Geometry check sheet. Reference: drawing and pictorial views, mm from the part's lowest x, y, z. Round coordinates to 2 decimals unless told otherwise and drop trailing zeros. Order: outer loops, then holes, each group sorted by start corner. A loop starts at its lowest first (then second) coordinate and runs counter-clockwise, first axis right, second up. Notation, with made-up numbers: (21.5, -5.5) -> (77.5, -5.5) arc R32 ccw to (77.5, 23.5) -> close; hole circle Ø10 at (36, 28.5). An arc over 180 degrees is marked (long way). Return JSON: item names as keys, results as strings. Group by question number.
1) Section check D-D on z = 1.7. Enter the section's corners in (x, y), plus the area to 3 significant figures.
2) Section check A-A on x = 3.25. Enter the section's corners in (y, z), plus the area to 3 significant figures.
3) Section check C-C on y = 0.85. Enter the section's corners in (x, z), plus the area to 3 significant figures.
4) Scan lines: L1, parallel to Z at x = 3.25, y = 0.35; L2, parallel to X at y = 0.3, z = 3.6; L3, parallel to X at y = 0.1, z = 1.85. Record each from-to range of solid material in increasing order.
5) Draft check along X on the marked faces 1 and 2. Enter one of: pulls with the +X half, pulls with the -X half, needs draft (parallel to the pull), parting line crosses it, or undercut.
6) Section check B-B on z = 2.8. Enter the section's corners in (x, y).
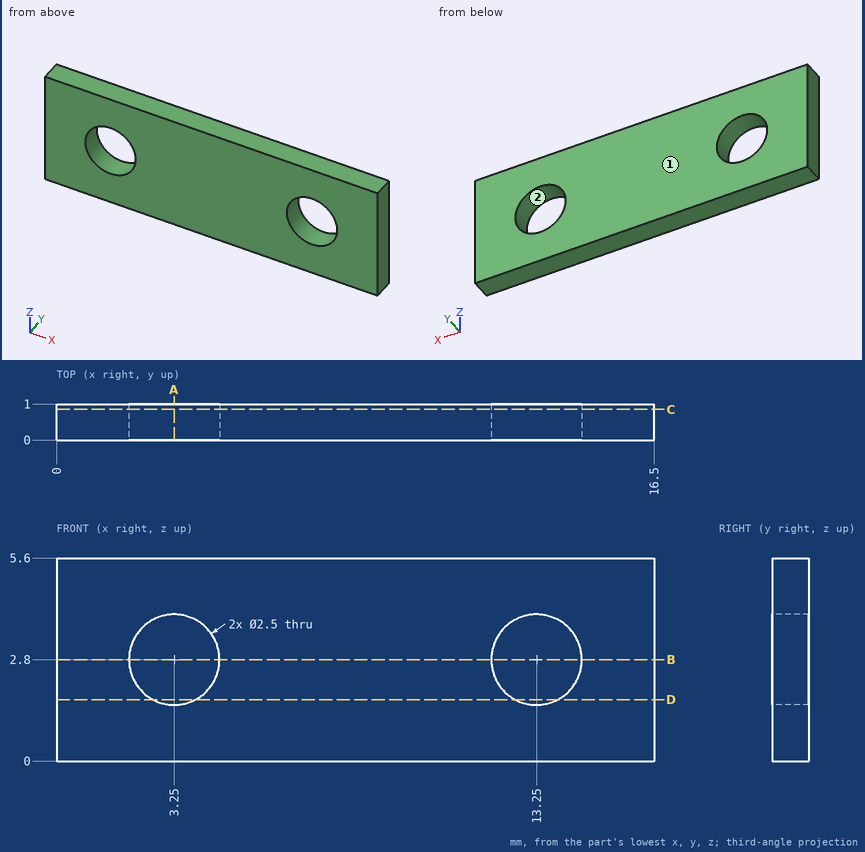
Check result:
{
 "1": {"outline": "(0, 0) -> (2.66, 0) -> (2.66, 1) -> (0, 1) -> close; (3.84, 0) -> (12.66, 0) -> (12.66, 1) -> (3.84, 1) -> close; (13.84, 0) -> (16.5, 0) -> (16.5, 1) -> (13.84, 1) -> close", "area": "14.1 mm^2"},
 "2": {"outline": "(0, 0) -> (1, 0) -> (1, 1.55) -> (0, 1.55) -> close; (0, 4.05) -> (1, 4.05) -> (1, 5.6) -> (0, 5.6) -> close", "area": "3.10 mm^2"},
 "3": {"outline": "(0, 0) -> (16.5, 0) -> (16.5, 5.6) -> (0, 5.6) -> close; hole circle Ø2.5 at (3.25, 2.8); hole circle Ø2.5 at (13.25, 2.8)", "area": "82.6 mm^2"},
 "4": {"L1": "0 to 1.55, 4.05 to 5.6", "L2": "0 to 2.29, 4.21 to 12.29, 14.21 to 16.5", "L3": "0 to 2.44, 4.06 to 12.44, 14.06 to 16.5"},
 "5": {"face 1": "needs draft", "face 2": "undercut"},
 "6": {"outline": "(0, 0) -> (2, 0) -> (2, 1) -> (0, 1) -> close; (4.5, 0) -> (12, 0) -> (12, 1) -> (4.5, 1) -> close; (14.5, 0) -> (16.5, 0) -> (16.5, 1) -> (14.5, 1) -> close"}
}
